from build123d import *

# Parameters (mm, degrees)
BOSS_EXTRUDE1_DEPTH             = 3
SKETCH2_W                       = 30
SKETCH2_H                       = 3
BOSS_EXTRUDE2_DEPTH             = 44
BOSS_EXTRUDE2_DIRECTION_2_REACH = 76.018
SKETCH3_R                       = 1
CUT_EXTRUDE1_DEPTH              = 10
SKETCH5_R                       = 4.5
SKETCH5_R_2                     = 1.05
CUT_EXTRUDE2_DEPTH              = 90.56424105


with BuildPart() as part:
    # Sketch1 → Boss-Extrude1 (new body)
    with BuildSketch(Plane(origin=(0, 0, 0), x_dir=(1, 0, 0), z_dir=(0, 1, 0))):
        with BuildLine():
            ThreePointArc((-52.563656192, 11.590548397), (-53.910964998, 14.843239591), (-57.163656192, 16.190548397))
            Line((-57.163656192, 16.190548397), (-57.163656192, 14.190548397))
            ThreePointArc((-57.163656192, 14.190548397), (-55.32517856, 13.429026028), (-54.563656192, 11.590548397))
            ThreePointArc((-54.563656192, 11.590548397), (-55.32517856, 9.752070766), (-57.163656192, 8.990548397))
            Line((-57.163656192, 8.990548397), (-57.163656192, 6.990548397))
            ThreePointArc((-57.163656192, 6.990548397), (-53.910964998, 8.337857204), (-52.563656192, 11.590548397))
        make_face()
        with BuildLine():
            Line((-57.163656192, 14.190548397), (-57.163656192, 16.190548397))
            ThreePointArc((-57.163656192, 16.190548397), (-60.416347385, 14.843239591), (-61.763656192, 11.590548397))
            ThreePointArc((-61.763656192, 11.590548397), (-60.416347385, 8.337857204), (-57.163656192, 6.990548397))
            Line((-57.163656192, 6.990548397), (-57.163656192, 8.990548397))
            ThreePointArc((-57.163656192, 8.990548397), (-59.763656192, 11.590548397), (-57.163656192, 14.190548397))
        make_face()
        with BuildLine():
            ThreePointArc((-42.163656192, -8.409451603), (-49.808275889, 0.319346154), (-52.563656192, 11.590548397))
            ThreePointArc((-52.563656192, 11.590548397), (-53.910964998, 8.337857204), (-57.163656192, 6.990548397))
            Line((-57.163656192, 6.990548397), (-57.163656192, -8.409451603))
            Line((-57.163656192, -8.409451603), (-42.163656192, -8.409451603))
        make_face()
        with BuildLine():
            ThreePointArc((-57.163656192, 6.990548397), (-60.416347385, 8.337857204), (-61.763656192, 11.590548397))
            ThreePointArc((-61.763656192, 11.590548397), (-64.519036494, 0.319346154), (-72.163656192, -8.409451603))
            Line((-72.163656192, -8.409451603), (-57.163656192, -8.409451603))
            Line((-57.163656192, -8.409451603), (-57.163656192, 6.990548397))
        make_face()
    extrude(amount=-BOSS_EXTRUDE1_DEPTH)

    # Sketch2 → Boss-Extrude2 (add)
    with BuildSketch(Plane(origin=(0, -3, 0), x_dir=(-1, 0, 0), z_dir=(0, -1, 0))):
        with Locations((57.163656192, -9.909451603)):
            Rectangle(SKETCH2_W, SKETCH2_H)
    extrude(amount=BOSS_EXTRUDE2_DEPTH)

    # Boss-Extrude2 direction 2: up to this face of the body (flat: up to its plane)
    boss_extrude2_direction_2_end = Plane(part.part.faces().sort_by_distance((-57.163656192, 0, -0.136432956))[0])
    # Sketch2 → Boss-Extrude2 direction 2 (add, up to the picked face)
    with BuildSketch(Plane(origin=(0, -3, 0), x_dir=(-1, 0, 0), z_dir=(0, -1, 0)), mode=Mode.PRIVATE) as boss_extrude2_direction_2_sk1:
        with Locations((57.163656192, -9.909451603)):
            Rectangle(SKETCH2_W, SKETCH2_H)
    boss_extrude2_direction_2_tool1 = split(extrude(boss_extrude2_direction_2_sk1.sketch, amount=-BOSS_EXTRUDE2_DIRECTION_2_REACH, mode=Mode.PRIVATE), bisect_by=boss_extrude2_direction_2_end, keep=Keep.BOTH, mode=Mode.PRIVATE)
    add(boss_extrude2_direction_2_tool1.solids().sort_by(Axis((-57.163656, -3, 9.909452), (0, 1, 0)))[0])

    # Sketch3 → Cut-Extrude1 (cut)
    with BuildSketch(Plane(origin=(0, -47, 0), x_dir=(-1, 0, 0), z_dir=(0, -1, 0))):
        with Locations(Location((47.163656192, -9.909451603, 0), (0, 0, 90))):
            Circle(SKETCH3_R)
        with Locations(Location((67.163656192, -9.909451603, 0), (0, 0, 90))):
            Circle(SKETCH3_R)
    extrude(amount=-CUT_EXTRUDE1_DEPTH, mode=Mode.SUBTRACT)

    # Sketch5 → Cut-Extrude2 (cut, through all)
    with BuildSketch(Plane(origin=(0, 0, 8.409451603), x_dir=(-1, 0, 0), z_dir=(0, 0, -1))):
        with Locations((57.163656192, -13)):
            Circle(SKETCH5_R)
        with Locations((52.353656192, -7.485)):
            Circle(SKETCH5_R_2)
        with Locations((52.353656192, -18.515)):
            Circle(SKETCH5_R_2)
        with Locations((61.973656192, -7.485)):
            Circle(SKETCH5_R_2)
        with Locations((61.973656192, -18.515)):
            Circle(SKETCH5_R_2)
    extrude(amount=-CUT_EXTRUDE2_DEPTH, mode=Mode.SUBTRACT)


solid = part.part
Model file for the job. Use its own axes, mm. A direction names the side the tool comes from. Give positions to 0.01 mm unless a question says otherwise; leave off trailing zeros. Loops run counter-clockwise (first coordinate to the right, second up) from the corner with the lowest first, then second, coordinate; pieces in that order, holes last.
1) Tool access for faces 1 (the flat face through (-47, -37, 10)), 2 (the flat face through (-57, -25, 8.409)), 3 (the flat face through (-57, -24, 11.409)): list every direction of +Z, -Z, +X, -X, +Y, -Y with a clear straight run to the whole face (end or side of a thin tool).
2) Saw through at D-D (y = -21). Write the cut outline in (x, z), plus the area to 3 significant figures.
3) Wall check: line 1 (Z direction, x = -69, y = -21); line 2 (Y direction, x = -61.5, z = -8.75); line 3 (X direction, y = -12, z = 9.75). Give the ranges that are in metal, low to high.
4) Flat gauge pins, fed straight in: pin 1 Ø8 at (x, z) = (-48.5, -8) entering from -Y; pin 2 Ø4 at (x, y) = (-67.5, -9) entering from -Z; pin 3 Ø0.6 at (x, z) = (-47, 9.5) entering from -Y. Where does each tip first touch, or does it go through?
5) Saw through at A-A (y = -10). Write the cut outline in (x, z).
6) Saw through at B-B (z = -10.25). Write the cut outline in (x, y).
7) Pull direction Y, two halves, no side cores. Call faces 4 (the cylindrical face through (-52.67, -12.8, 9.89)), 5 (the cylindrical face through (-46.32, -42.07, 9.37)), 6 (the flat face through (-57, -3, -1)): +Y half, -Y half, draft (parallel to the pull), parting line (faces both ways), or undercut.
8) Saw through at C-C (x = -52). Write the cut outline in (y, z), plus the area to 3 significant figures.
Answer block:
1. face 1: -Y
1. face 2: -Z, +X, -X, -Y
1. face 3: +Z, +X, -X, +Y, -Y
2. outline: (-72.16, 8.41) - (-42.16, 8.41) - (-42.16, 11.41) - (-72.16, 11.41) - close
2. area: 90.0 mm2
3. line 1: z = 8.41 to 11.41
3. line 2: y = -3 to 0
3. line 3: x = -72.16 to -61.55, -52.78 to -42.16
4. pin 1: stops at y = -3
4. pin 2: stops at z = 8.41
4. pin 3: stops at y = -37
5. outline: (-72.16, 8.41) - (-60.52, 8.41) - (-60.52, 11.41) - (-72.16, 11.41) - close; (-53.81, 8.41) - (-42.16, 8.41) - (-42.16, 11.41) - (-53.81, 11.41) - close
6. outline: (-61.8, -3) - (-59.39, -3) - (-59.39, 0) - (-61.8, 0) - close; (-54.94, -3) - (-52.53, -3) - (-52.53, 0) - (-54.94, 0) - close
7. face 4: undercut
7. face 5: draft
7. face 6: -Y half
8. outline: (-47, 8.41) - (-19.5, 8.41) - (-19.5, 11.41) - (-47, 11.41) - close; (-17.53, 8.41) - (-8.47, 8.41) - (-8.47, 11.41) - (-17.53, 11.41) - close; (-6.5, 8.41) - (-3, 8.41) - (-3, -6.37) - (0, -6.37) - (0, 11.41) - (-6.5, 11.41) - close
8. area: 173 mm2
